Design review of the part built by this model. Coordinates are the model's own, in mm. Face numbers are marked on the shaded views. A direction names the side the tool comes from. Round coordinates to 2 decimals unless told otherwise and drop trailing zeros. Write each loop counter-clockwise with the first axis right and the second up, starting at its lowest first coordinate (ties: lowest second). Pieces come first, ordered by that corner, then holes. Notation, with made-up numbers: M 9.5,33 L 68.5,33 A32 ccw 68.5,68 Z; hole C 70,6 d3. An arc over 180 degrees is marked long. One line per question, with ' | ' between items. Start each with the question number.
Item 1: Add section D-D, the plane y = 1.2. State the section outline as (x, z) points (3 decimals), and give its area (3 significant figures).
Item 2: For L1, parallel to Z at x = 4, y = -0.15 (3 decimals); L2, parallel to Y at x = 0, z = 3.1; L3, parallel to X at y = -0.5, z = 2.75, list the stretches that pass through material, from the lowest coordinate up.
Item 3: Add section A-A, the plane y = 0. State the section outline as (x, z) points (3 decimals), and give its area (3 significant figures).
Item 4: Draft analysis for pull direction Z (two halves, no side actions). For the marked faces 1, 2 and 3, state which applies: released by +Z, released by -Z, zero draft, split by the parting line, or undercut.
Item 5: Add section B-B, the plane z = 1.8. State the section outline as (x, y) points, and give its area (3 significant figures).
Item 6: Machinability: for the marked faces 4 and 5, which of the approach directions +Z, -Z, +X, -X, +Y, -Y give a long, thin tool a straight path to every point of the face, cutting with its end or side? Answer none if there is none.
Item 7: Add section C-C, the plane x = 0. State the section outline as (y, z) points (3 decimals).
```python
from build123d import *

# Parameters (mm, degrees)
SKETCH1_R           = 0.75
BOSS_EXTRUDE1_DEPTH = 0.5
SKETCH2_R           = 1.651
SKETCH2_R_2         = 0.75
BOSS_EXTRUDE2_DEPTH = 3.175


with BuildPart() as part:
    # Sketch1 → Boss-Extrude1 (new body)
    with BuildSketch(Plane.XY):
        with BuildLine():
            ThreePointArc((0.835526316, 2.356246119), (-2.5, 0), (0.835526316, -2.356246119))
            ThreePointArc((0.835526316, -2.356246119), (3.175, -1.953735254), (5.514473684, -2.356246119))
            ThreePointArc((5.514473684, -2.356246119), (8.85, 0), (5.514473684, 2.356246119))
            ThreePointArc((5.514473684, 2.356246119), (3.175, 1.953735254), (0.835526316, 2.356246119))
        make_face()
        Circle(SKETCH1_R, mode=Mode.SUBTRACT)
        with Locations(Location((6.35, 0, 0), (0, 0, 180))):
            Circle(SKETCH1_R, mode=Mode.SUBTRACT)
    extrude(amount=BOSS_EXTRUDE1_DEPTH)

    # Sketch2 → Boss-Extrude2 (add)
    # profile 1 of 2: a face of its own
    with BuildSketch(Plane.XY.offset(0.5)):
        with Locations((6.35, 0)):
            Circle(SKETCH2_R)
        with Locations(Location((6.35, 0, 0), (0, 0, 180))):
            Circle(SKETCH2_R_2, mode=Mode.SUBTRACT)
    # profile 2 of 2: a face of its own
    with BuildSketch(Plane.XY.offset(0.5)):
        Circle(SKETCH2_R)
        Circle(SKETCH2_R_2, mode=Mode.SUBTRACT)
    extrude(amount=BOSS_EXTRUDE2_DEPTH)

    # Mirror1: part across plane


with BuildPart() as part_1:
    add(part.part)
    add(part.part.mirror(Plane.XY.offset(2.0875)))


solid = part_1.part
```
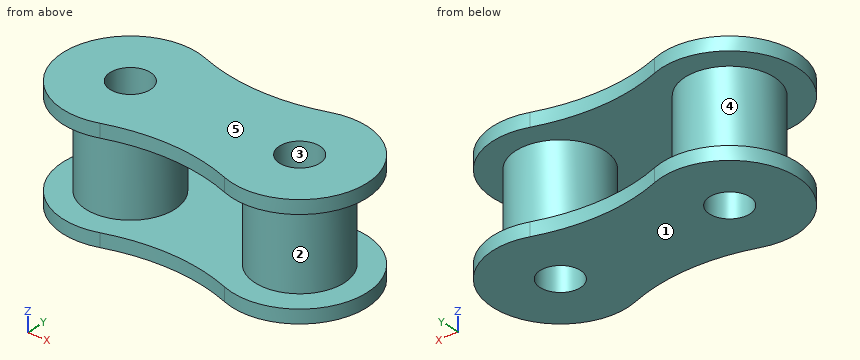
Computed values:
1) outline: M -2.193,0 L 8.543,0 L 8.543,0.5 L 7.484,0.5 L 7.484,3.675 L 8.543,3.675 L 8.543,4.175 L -2.193,4.175 L -2.193,3.675 L -1.134,3.675 L -1.134,0.5 L -2.193,0.5 Z; hole M 1.134,0.5 L 5.216,0.5 L 5.216,3.675 L 1.134,3.675 Z | area: 25.1 mm^2
2) L1: z = 0 to 0.5, 3.675 to 4.175 | L2: y = -1.65 to -0.75, 0.75 to 1.65 | L3: x = -1.57 to -0.56, 0.56 to 1.57, 4.78 to 5.79, 6.91 to 7.92
3) outline: M -2.5,0 L -0.75,0 L -0.75,4.175 L -2.5,4.175 L -2.5,3.675 L -1.651,3.675 L -1.651,0.5 L -2.5,0.5 Z; M 0.75,0 L 5.6,0 L 5.6,4.175 L 0.75,4.175 Z; M 7.1,0 L 8.85,0 L 8.85,0.5 L 8.001,0.5 L 8.001,3.675 L 8.85,3.675 L 8.85,4.175 L 7.1,4.175 Z; hole M 1.651,0.5 L 4.699,0.5 L 4.699,3.675 L 1.651,3.675 Z | area: 19.8 mm^2
4) face 1: released by -Z | face 2: undercut | face 3: zero draft
5) outline: C 0,0 d3.3; C 6.35,0 d3.3; hole C 0,0 d1.5; hole C 6.35,0 d1.5 | area: 13.6 mm^2
6) face 4: none | face 5: +Z, +X, -X, +Y, -Y
7) outline: M -2.5,0 L -0.75,0 L -0.75,4.175 L -2.5,4.175 L -2.5,3.675 L -1.651,3.675 L -1.651,0.5 L -2.5,0.5 Z; M 0.75,0 L 2.5,0 L 2.5,0.5 L 1.651,0.5 L 1.651,3.675 L 2.5,3.675 L 2.5,4.175 L 0.75,4.175 Z
